Work out the finished part from the listing and answer in its coordinate system (mm). Face numbers are marked on the shaded views. A direction names the side the tool comes from. Round coordinates to 2 decimals unless told otherwise and drop trailing zeros. Loops run counter-clockwise (first coordinate to the right, second up) from the corner with the lowest first, then second, coordinate; pieces in that order, holes last. Notation, with made-up numbers: (34.5, 69.5) - (85.5, 69.5) arc R14 cw to (85.5, 88.5) - close; hole circle Ø4 at (60.5, -37.75). An arc over 180 degrees is marked (long way). Answer as CSV lines item,"result". Start each with the question number.
Q1. The mould has two halves that part along Y. Classify the marked faces 1, 2 and 3: +Y half, -Y half, draft (parallel to the pull), parting line (faces both ways), or undercut.
Q2. Section C-C on x = -17 is taken. Write down the section's boundary in (y, z), then the cut area to 3 significant figures.
Q3. For the marked faces 4, 5, 6, 7 and 8, determine the directions among +Z, -Z, +X, -X, +Y, -Y from which every point of the face is accessible in a straight line to the end or side of a thin tool.
Q4. Each of these flat-tipped pins is pushed along its axis until it touches: pin 1 Ø12 at (y, z) = (24.5, -8) entering from +X; pin 2 Ø5 at (x, z) = (-9, 2.5) entering from -Y; pin 3 Ø2 at (x, y) = (-14.5, -6) entering from +Z; pin 4 Ø1.3 at (x, z) = (10.5, -4) entering from -Y. Where does it stop, or does it pass through?
Q5. Section A-A on y = -18 is taken. Write down the section's boundary in (x, z).
Q6. Straight lines are drawn through the part: L1, parallel to Y at x = 2.75, z = 0; L2, parallel to X at y = -15.5, z = 8.5; L3, parallel to Y at x = 18.5, z = 0. For each, find the intervals that lie inside material, in ascending order. Write a range as [from, to].
Q7. Section D-D on z = 16.5 is taken. Write down the section's boundary in (x, y).
Q8. Section B-B on y = 22 is taken. Write down the section's boundary in (x, z).
```python
from build123d import *

# Parameters (mm, degrees)
SKETCH1_R           = 22.5
BOSS_EXTRUDE1_DEPTH = 3
SKETCH2_R           = 5
BOSS_EXTRUDE2_DEPTH = 70
SKETCH3_R           = 12
BOSS_EXTRUDE3_DEPTH = 28
FILLET1_R           = 6
SKETCH4_W           = 20
SKETCH4_H           = 20
CUT_EXTRUDE1_DEPTH  = 14
SKETCH6_R           = 5
CUT_EXTRUDE2_DEPTH  = 31
SKETCH7_R           = 9
SKETCH7_R_2         = 5
BOSS_EXTRUDE4_DEPTH = 12.5


with BuildPart() as part:
    # Sketch1 → Boss-Extrude1 (new body)
    with BuildSketch(Plane(origin=(0, 0, 0), x_dir=(1, 0, 0), z_dir=(0, 1, 0))):
        Circle(SKETCH1_R)
    extrude(amount=BOSS_EXTRUDE1_DEPTH)

    # Sketch2 → Boss-Extrude2 (add)
    with BuildSketch(Plane(origin=(0, 3, 0), x_dir=(1, 0, 0), z_dir=(0, 1, 0))):
        Circle(SKETCH2_R)
    extrude(amount=BOSS_EXTRUDE2_DEPTH)

    # Sketch3 → Boss-Extrude3 (add)
    with BuildSketch(Plane.XZ):
        Circle(SKETCH3_R)
    extrude(amount=BOSS_EXTRUDE3_DEPTH)

    # Fillet1
    fillet1_edges = [part.edges().sort_by_distance(p)[0] for p in [
        (-12, -28, 0),
    ]]
    fillet(fillet1_edges, radius=FILLET1_R)

    # Sketch4 → Cut-Extrude1 (cut, symmetric)
    with BuildSketch(Plane.XY):
        with Locations((17.5, -18)):
            Rectangle(SKETCH4_W, SKETCH4_H)
        with Locations((-17.5, -18)):
            Rectangle(SKETCH4_W, SKETCH4_H)
    extrude(amount=CUT_EXTRUDE1_DEPTH, both=True, mode=Mode.SUBTRACT)

    # Sketch6 → Cut-Extrude2 (cut, through all)
    with BuildSketch(Plane(origin=(7.5, 0, 0), x_dir=(0, 0, -1), z_dir=(1, 0, 0))):
        with Locations((0, -18)):
            Circle(SKETCH6_R)
    extrude(amount=-CUT_EXTRUDE2_DEPTH, mode=Mode.SUBTRACT)

    # Sketch7 → Boss-Extrude4 (add, symmetric)
    with BuildSketch(Plane(origin=(0, 0, 0), x_dir=(0, 0, -1), z_dir=(1, 0, 0))):
        with Locations((0, -18)):
            Circle(SKETCH7_R)
        with Locations((0, -18)):
            Circle(SKETCH7_R_2, mode=Mode.SUBTRACT)
    extrude(amount=BOSS_EXTRUDE4_DEPTH, both=True)


solid = part.part
```
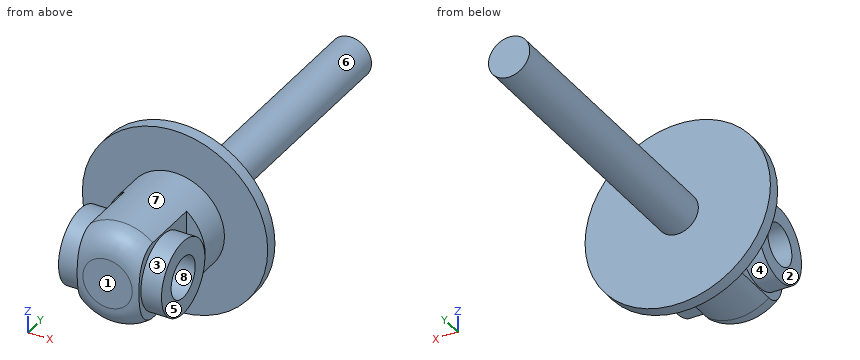
Findings:
1,face 1,"-Y half"
1,face 2,"draft"
1,face 3,"undercut"
2,outline,"(0, -14.74) - (3, -14.74) - (3, 14.74) - (0, 14.74) - close"
2,area,"88.4 mm^2"
3,face 4,"-X"
3,face 5,"+Z, -Z, +X, -Y"
3,face 6,"+Y"
3,face 7,"none"
3,face 8,"+X, -X"
4,pin 1,"stops at x = 4.58"
4,pin 2,"stops at y = -27.94"
4,pin 3,"passes through"
4,pin 4,"stops at y = -26.35"
5,outline,"(-12.5, -9) - (-7.5, -9) - (-7.5, -9.37) arc R12 ccw to (7.5, -9.37) - (7.5, -9) - (12.5, -9) - (12.5, -5) - (-12.5, -5) - close; (-12.5, 5) - (12.5, 5) - (12.5, 9) - (7.5, 9) - (7.5, 9.37) arc R12 ccw to (-7.5, 9.37) - (-7.5, 9) - (-12.5, 9) - close"
6,L1,"y = [-28, -23], [-13, 73]"
6,L2,"x = [-12.5, 12.5]"
6,L3,"y = [0, 3]"
7,outline,"(-15.3, 0) - (15.3, 0) - (15.3, 3) - (-15.3, 3) - close"
8,outline,"circle Ø10 at (0, 0)"
